Autodesk Inventor part; units mm, degrees
ref_plane "YZ Plane" through (0, 0, 0) normal (1, 0, 0) x (0, 1, 0)
ref_plane "XZ Plane" through (0, 0, 0) normal (0, 1, 0) x (-1, 0, 0)
ref_plane "XY Plane" through (0, 0, 0) normal (0, 0, 1) x (1, 0, 0)
sketch "Sketch1" plane through (0, 0, 0) normal (0, 0, 1) x (1, 0, 0)
  line L0 (0, 0) -> (-50.8, 0)
  line L1 (-50.8, 0) -> (-50.8, -25.4)
  line L2 (-50.8, -25.4) -> (0, -25.4)
  line L3 (0, -25.4) -> (0, 0)
  line L4 (-3.175, -22.225) -> (-47.625, -22.225)
  line L5 (-47.625, -22.225) -> (-47.625, -3.175)
  line L6 (-47.625, -3.175) -> (-3.175, -3.175)
  line L7 (-3.175, -3.175) -> (-3.175, -22.225)
  dimension "d0" = 50.8
  dimension "d1" = 25.4
  dimension "d2" = 3.175
extrude "Extrusion1" add sketch "Sketch1" along normal blind 228.6
sketch "Sketch2" plane through (-50.8, -25.4, 0) normal (0, -1, 0) x (1, 0, 0)
  line L0 (0, 228.6) -> (50.8, 228.6)
  line L1 (50.8, 228.6) -> (25.4, 228.6)
  line L2 (25.4, 228.6) -> (25.4, 88.9)
  line L3 (25.4, 88.9) -> (50.8, 88.9)
  line L4 (50.8, 88.9) -> (50.8, 228.6)
  point P0 (50.8, 0)
  dimension "d5" = 25.4
  dimension "d6" = 139.7
extrude "Extrusion2" cut sketch "Sketch2" against normal blind 25.4
sketch "Sketch3" plane through (-50.8, -25.4, 0) normal (0, -1, 0) x (1, 0, 0)
  circle A0 centre (12.7, 215.9) radius 3.3734
  circle A1 centre (12.7, 190.5) radius 3.3734
  line L0 (25.4, 88.9) -> (25.4, 228.6)
  line L1 (0, 228.6) -> (25.4, 228.6)
  point P0 (50.8, 0)
  dimension "d9" = 6.7469
  dimension "d10" = 6.7469
  dimension "d11" = 12.7
  dimension "d12" = 12.7
  dimension "d13" = 12.7
  dimension "d14" = 38.1
extrude "Extrusion3" cut sketch "Sketch3" against normal blind 25.4
sketch "Sketch4" plane through (-50.8, 0, 0) normal (0, 1, 0) x (1, 0, 0)
  circle A0 centre (12.7, -50.8) radius 3.3734
  circle A1 centre (12.7, -76.2) radius 3.3782
  line L0 (50.8, 0) -> (0, 0)
  line L1 (0, 0) -> (0, -228.6)
  dimension "d17" = 6.7469
  dimension "d18" = 6.7564
  dimension "d19" = 50.8
  dimension "d20" = 12.7
  dimension "d21" = 12.7
  dimension "d22" = 25.4
extrude "Extrusion4" cut sketch "Sketch4" against normal blind 25.4
properties part number "vertical support" material "Aluminum 6061"
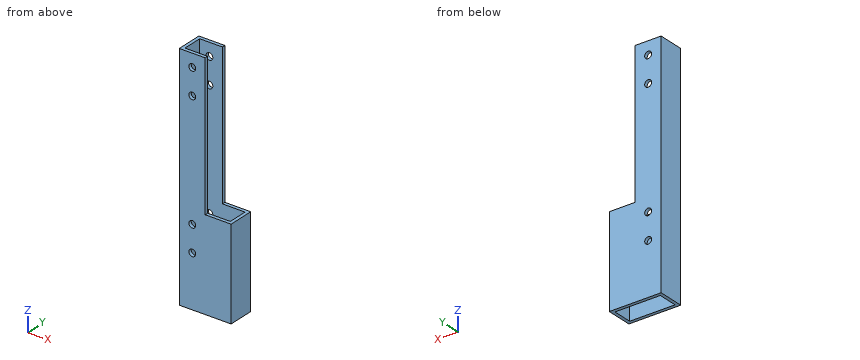
The model under review builds one solid part; all positions refer to its coordinate system, in mm. Coordinates: 2 decimals unless noted, no trailing zeros. Write each loop counter-clockwise with the first axis right and the second up, starting at its lowest first coordinate (ties: lowest second). Pieces come first, ordered by that corner, then holes. Notation, with made-up numbers: (74, -30.5) -> (131, -30.5) arc R25 ccw to (131, -3.5) -> close; hole circle Ø5 at (44.25, 11.5). An arc over 180 degrees is marked (long way). Answer in a Markdown table with one row per item.
1. We need section B-B, the plane z = 215.9. State the section outline as (x, y) points (3 decimals), and give its area (3 significant figures).
Answers below:
| item | result |
|---|---|
| outline | (-50.8, -25.4) -> (-41.473, -25.4) -> (-41.473, -22.225) -> (-47.625, -22.225) -> (-47.625, -3.175) -> (-41.473, -3.175) -> (-41.473, 0) -> (-50.8, 0) -> close; (-34.727, -25.4) -> (-25.4, -25.4) -> (-25.4, -22.225) -> (-34.727, -22.225) -> close; (-34.727, -3.175) -> (-25.4, -3.175) -> (-25.4, 0) -> (-34.727, 0) -> close |
| area | 179 mm^2 |
2. We need section A-A, the plane z = 50.8. State the section outline as (x, y) points (3 decimals).
Answers below:
| item | result |
|---|---|
| outline | (-50.8, -25.4) -> (-41.473, -25.4) -> (-41.473, -22.225) -> (-47.625, -22.225) -> (-47.625, -3.175) -> (-41.473, -3.175) -> (-41.473, 0) -> (-50.8, 0) -> close; (-34.727, -25.4) -> (0, -25.4) -> (0, 0) -> (-34.727, 0) -> (-34.727, -3.175) -> (-3.175, -3.175) -> (-3.175, -22.225) -> (-34.727, -22.225) -> close |
3. Wall thickness on probe 1 along Z at (x, y) = (-38.1, -24.05); probe 2 along X at (y, z) = (-23.7, 50.8); probe 3 along Y at (x, z) = (-25, 82.5) (3 decimals): over which ranges is each line inside the solid? List them lowest first. Write a range as [from, to].
Answers below:
| item | result |
|---|---|
| probe 1 | z = [0, 47.43], [54.17, 72.82], [79.58, 187.13], [193.87, 212.53], [219.27, 228.6] |
| probe 2 | x = [-50.8, -41.47], [-34.73, 0] |
| probe 3 | y = [-25.4, -22.225], [-3.175, 0] |
4. We need section D-D, the plane y = -7.25. State the section outline as (x, z) points (3 decimals), and give its area (3 significant figures).
Answers below:
| item | result |
|---|---|
| outline | (-50.8, 0) -> (-47.625, 0) -> (-47.625, 228.6) -> (-50.8, 228.6) -> close; (-3.175, 0) -> (0, 0) -> (0, 88.9) -> (-3.175, 88.9) -> close |
| area | 1,010 mm^2 |
5. Clearance check with flat-ended pins moving along their axes: pin 1 Ø4 at (y, z) = (-11, 188) entering from +X (3 decimals); pin 2 Ø4 at (x, z) = (-38.1, 190.5) entering from -Y; pin 3 Ø3.5 at (y, z) = (-1, 171.5) entering from +X. State where each tip first meets the part, or that it passes through.
Answers below:
| item | result |
|---|---|
| pin 1 | stops at x = -47.625 |
| pin 2 | passes through |
| pin 3 | stops at x = -25.4 |
6. We need section C-C, the plane x = -16. State the section outline as (y, z) points (3 decimals).
Answers below:
| item | result |
|---|---|
| outline | (-25.4, 0) -> (-22.225, 0) -> (-22.225, 88.9) -> (-25.4, 88.9) -> close; (-3.175, 0) -> (0, 0) -> (0, 88.9) -> (-3.175, 88.9) -> close |
